Model file for the job. Use its own axes, mm. A direction names the side the tool comes from. Round coordinates to 2 decimals unless told otherwise and drop trailing zeros. Order: outer loops, then holes, each group sorted by start corner. A loop starts at its lowest first (then second) coordinate and runs counter-clockwise, first axis right, second up. Notation, with made-up numbers: (-37, -10) - (-19, -10) arc R25 cw to (-19, 10) - close; hole circle Ø4 at (-1.5, -39.5). An arc over 180 degrees is marked (long way). Write item = value, one per line.
```python
from build123d import *

# Parameters (mm, degrees)
SKETCH2_W                                           = 150
SKETCH2_H                                           = 30
BOSS_EXTRUDE1_DEPTH                                 = 30
SKETCH3_R                                           = 13.75
CUT_EXTRUDE1_DEPTH                                  = 23
LPATTERN1_COUNT                                     = 5
LPATTERN1_PITCH                                     = 30
CBORE_FOR_M4_HEX_SOCKET_HEAD_CAP_SCREW1_D           = 4.5
CBORE_FOR_M4_HEX_SOCKET_HEAD_CAP_SCREW1_CBORE_D     = 8
CBORE_FOR_M4_HEX_SOCKET_HEAD_CAP_SCREW1_CBORE_DEPTH = 4.4
LPATTERN2_COUNT                                     = 2
LPATTERN2_PITCH                                     = 120
SKETCH7_W                                           = 181.12901383
SKETCH7_H                                           = 4
CUT_EXTRUDE3_DEPTH                                  = 23
SKETCH8_W                                           = 4
SKETCH8_H                                           = 50
CUT_EXTRUDE4_DEPTH                                  = 23
SKIZZE1_R                                           = 16
SKIZZE1_R_2                                         = 15
SCHNITT_LINEAR_AUSTRAGEN1_DEPTH                     = 80.868642157
LPATTERN3_COUNT                                     = 5
LPATTERN3_PITCH                                     = 30
CBORE_FOR_M6_HEX_SOCKET_HEAD_CAP_SCREW1_D           = 6.6
CBORE_FOR_M6_HEX_SOCKET_HEAD_CAP_SCREW1_CBORE_D     = 11
CBORE_FOR_M6_HEX_SOCKET_HEAD_CAP_SCREW1_CBORE_DEPTH = 4.4
LPATTERN4_COUNT                                     = 2
LPATTERN4_PITCH                                     = 75


with BuildPart() as part:
    # Sketch2 → Boss-Extrude1 (new body)
    with BuildSketch(Plane(origin=(0, 0, 0), x_dir=(1, 0, 0), z_dir=(0, 1, 0))):
        Rectangle(SKETCH2_W, SKETCH2_H)
    extrude(amount=BOSS_EXTRUDE1_DEPTH)

    # Sketch3 → Cut-Extrude1 (cut)
    with BuildSketch(Plane(origin=(0, 30, 0), x_dir=(1, 0, 0), z_dir=(0, 1, 0))):
        with Locations(Location((-60, 0, 0), (0, 0, 270))):
            Circle(SKETCH3_R)
    cut_extrude1 = extrude(amount=-CUT_EXTRUDE1_DEPTH, mode=Mode.SUBTRACT)

    # LPattern1: Cut-Extrude1 ×5
    with Locations(*[(i * LPATTERN1_PITCH, 0, 0) for i in range(1, LPATTERN1_COUNT)]):
        add(cut_extrude1, mode=Mode.SUBTRACT)

    # CBORE for M4 Hex Socket Head Cap Screw1 (through all)
    with Locations(Plane(origin=(0, 7, 0), x_dir=(-1, 0, 0), z_dir=(0, 1, 0))):
        with Locations((60, 0)):
            cbore_for_m4_hex_socket_head_cap_screw1 = CounterBoreHole(CBORE_FOR_M4_HEX_SOCKET_HEAD_CAP_SCREW1_D / 2, CBORE_FOR_M4_HEX_SOCKET_HEAD_CAP_SCREW1_CBORE_D / 2, CBORE_FOR_M4_HEX_SOCKET_HEAD_CAP_SCREW1_CBORE_DEPTH)

    # LPattern2: CBORE for M4 Hex Socket Head Cap Screw1 ×2
    with Locations(*[(i * LPATTERN2_PITCH, 0, 0) for i in range(1, LPATTERN2_COUNT)]):
        add(cbore_for_m4_hex_socket_head_cap_screw1, mode=Mode.SUBTRACT)

    # Sketch7 → Cut-Extrude3 (cut)
    with BuildSketch(Plane(origin=(0, 30, 0), x_dir=(1, 0, 0), z_dir=(0, 1, 0))):
        Rectangle(SKETCH7_W, SKETCH7_H)
    extrude(amount=-CUT_EXTRUDE3_DEPTH, mode=Mode.SUBTRACT)

    # Sketch8 → Cut-Extrude4 (cut)
    with BuildSketch(Plane(origin=(0, 30, 0), x_dir=(-1, 0, 0), z_dir=(0, 1, 0))):
        with Locations((60, -1.298701607)):
            Rectangle(SKETCH8_W, SKETCH8_H)
    cut_extrude4 = extrude(amount=-CUT_EXTRUDE4_DEPTH, mode=Mode.SUBTRACT)

    # Skizze1 → Schnitt-Linear austragen1 (cut, through all)
    with BuildSketch(Plane(origin=(0, 7, 0), x_dir=(-1, 0, 0), z_dir=(0, 1, 0))):
        with Locations((60, 0)):
            Circle(SKIZZE1_R)
        with Locations((60, 0)):
            Circle(SKIZZE1_R_2, mode=Mode.SUBTRACT)
    schnitt_linear_austragen1 = extrude(amount=SCHNITT_LINEAR_AUSTRAGEN1_DEPTH, mode=Mode.SUBTRACT)

    # LPattern3: Cut-Extrude4, Schnitt-Linear austragen1 ×5
    with Locations(*[(i * LPATTERN3_PITCH, 0, 0) for i in range(1, LPATTERN3_COUNT)]):
        add(cut_extrude4, mode=Mode.SUBTRACT)
        add(schnitt_linear_austragen1, mode=Mode.SUBTRACT)

    # CBORE for M6 Hex Socket Head Cap Screw1 (through all)
    with Locations(Plane(origin=(0, 7, 0), x_dir=(-1, 0, 0), z_dir=(0, 1, 0))):
        with Locations((37.5, 0)):
            cbore_for_m6_hex_socket_head_cap_screw1 = CounterBoreHole(CBORE_FOR_M6_HEX_SOCKET_HEAD_CAP_SCREW1_D / 2, CBORE_FOR_M6_HEX_SOCKET_HEAD_CAP_SCREW1_CBORE_D / 2, CBORE_FOR_M6_HEX_SOCKET_HEAD_CAP_SCREW1_CBORE_DEPTH)

    # LPattern4: CBORE for M6 Hex Socket Head Cap Screw1 ×2
    with Locations(*[(i * LPATTERN4_PITCH, 0, 0) for i in range(1, LPATTERN4_COUNT)]):
        add(cbore_for_m6_hex_socket_head_cap_screw1, mode=Mode.SUBTRACT)


solid = part.part
```
1) Flat gauge pins, fed straight in: pin 1 Ø6.5 at (x, z) = (-37.5, 0) entering from -Y; pin 2 Ø1.5 at (x, z) = (39.5, -5.5) entering from +Y. Where does each tip first touch, or does it go through?
Conclusion:
pin_1 = through
pin_2 = 7
2) Wall check: line 1 along X through (y, z) = (1.25, -2); line 2 along Z through (x, y) = (-67.5, 21); line 3 along Z through (x, y) = (-37.5, 1.5). Give the ranges that are in metal, low to high.
Conclusion:
line_1 = -75 to -61.03, -58.97 to -40.12, -34.88 to 34.88, 40.12 to 58.97, 61.03 to 75
line_2 = -15 to -14.13, -12.99 to -11.52, 11.52 to 12.99, 14.13 to 15
line_3 = -15 to -3.3, 3.3 to 15
3) Cut at A-A (y = 4.25). Write the cut outline in (x, z), and give its area (3 significant figures).
Conclusion:
outline = (-75, -15) - (75, -15) - (75, 15) - (-75, 15) - close; hole circle Ø8 at (-60, 0); hole circle Ø11 at (-37.5, 0); hole circle Ø11 at (37.5, 0); hole circle Ø8 at (60, 0)
area = 4,210 mm^2
4) Cut at C-C (z = 0). Give the number of separate pieces and of enclosed holes in the cut face, and give its area (3 significant figures).
Conclusion:
separate_pieces = 5
enclosed_holes = 0
area = 825 mm^2
5) Cut at B-B (x = -60). Write the cut outline in (y, z), and give its area (3 significant figures).
Conclusion:
outline = (0, -15) - (7, -15) - (7, -4) - (2.6, -4) - (2.6, -2.25) - (0, -2.25) - close; (0, 2.25) - (2.6, 2.25) - (2.6, 4) - (7, 4) - (7, 15) - (0, 15) - close
area = 163 mm^2
6) 3-axis set-ups, long thin cutter, end or side, ignore diameter. For faces 1 (the face through (-70, 30, -10)), 2 (the face through (18.618, 18.339, 11.245)): which of +Z, -Z, +X, -X, +Y, -Y reach the whole face in a straight line?
Conclusion:
face_1 = +Z, -Z, +X, -X, +Y
face_2 = +Y
7) Mould opens along Z. For faces 3 (the face through (71.245, 18.339, 11.382)), 4 (the face through (-1, 5, -15)), 5 (the face through (72, 30, -12)) say: +Z half, -Z half, draft (parallel to the pull), parting line (faces both ways), or undercut.
Conclusion:
face_3 = undercut
face_4 = -Z half
face_5 = draft
